Geometry check sheet. Reference: drawing and pictorial views, mm from the part's lowest x, y, z. A direction names the side the tool comes from. Round coordinates to 2 decimals unless told otherwise and drop trailing zeros. Order: outer loops, then holes, each group sorted by start corner. A loop starts at its lowest first (then second) coordinate and runs counter-clockwise, first axis right, second up.
Q1. Cross-section at B-B on x = 13.75. Record the cut outline in (y, z), then the cut area to 3 significant figures.
Q2. Cross-section at A-A on z = 8. Record the cut outline in (x, y).
Q3. Set-up check for the marked faces 5, 6, 7, 8 and 9: record each of +Z, -Z, +X, -X, +Y, -Y from which the full face is reachable in a straight line by a thin tool's end or side.
Q4. Cross-section at C-C on x = 2.5. Record the cut outline in (y, z).
Q5. Scan lines: probe 1 along Y at (x, z) = (11.75, 12); probe 2 along X at (y, z) = (10.5, 4); probe 3 along Z at (x, y) = (11.75, 5.25). Record each from-to range of solid material in increasing order.
Q6. Depth check by flat-ended pin: P1, Ø0.6, axis at x = 16, y = 2.5, coming from the +Z side; P2, Ø0.6, axis at x = 11, y = 6.5, coming from the +Z side; P3, Ø2.5, axis at x = 5, z = 8.5, coming from the -Y side. Enter the tip coordinate at first touch or a pass-through.
Q7. Cross-section at D-D on z = 4.25. Record the cut outline in (x, y).
Q8. Mould release check, pull along X, two halves, no side actions. Record for the marked faces 1, 2, 3 and 4: +X half, -X half, draft (parallel to the pull), parting line (faces both ways), or undercut.
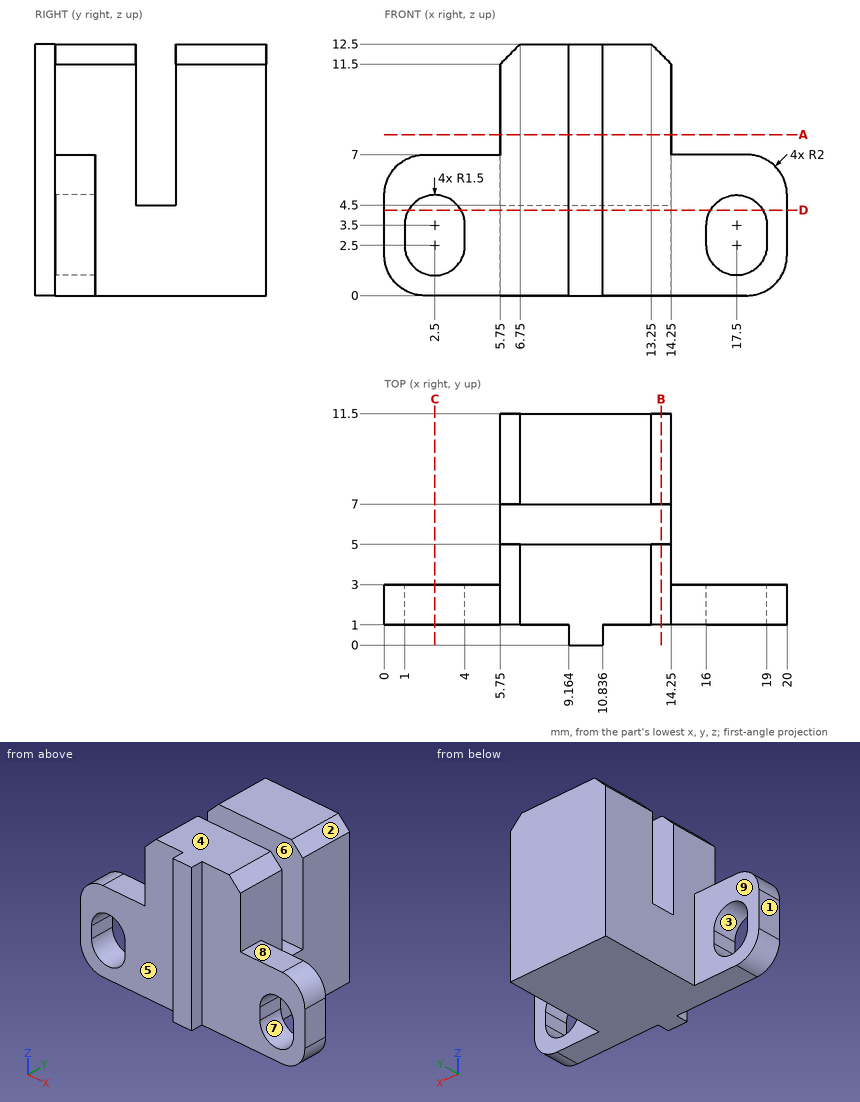
Results found:
1. outline: (1, 0) - (11.5, 0) - (11.5, 12) - (7, 12) - (7, 4.5) - (5, 4.5) - (5, 12) - (1, 12) - close
1. area: 111 mm2
2. outline: (5.75, 1) - (9.16, 1) - (9.16, 0) - (10.84, 0) - (10.84, 1) - (14.25, 1) - (14.25, 5) - (5.75, 5) - close; (5.75, 7) - (14.25, 7) - (14.25, 11.5) - (5.75, 11.5) - close
3. face 5: +Z, -Z, -X, -Y
3. face 6: +Z, +X, -X
3. face 7: +Y, -Y
3. face 8: +Z, +X, +Y, -Y
3. face 9: +Z, -Z, -X, +Y
4. outline: (1, 0) - (3, 0) - (3, 1) - (1, 1) - close; (1, 5) - (3, 5) - (3, 7) - (1, 7) - close
5. probe 1: y = 1 to 5, 7 to 11.5
5. probe 2: x = 5.75 to 14.25
5. probe 3: z = 0 to 4.5
6. P1: stops at z = 7
6. P2: stops at z = 4.5
6. P3: stops at y = 1
7. outline: (0, 1) - (1.2, 1) - (1.2, 3) - (0, 3) - close; (3.8, 1) - (9.16, 1) - (9.16, 0) - (10.84, 0) - (10.84, 1) - (16.2, 1) - (16.2, 3) - (14.25, 3) - (14.25, 11.5) - (5.75, 11.5) - (5.75, 3) - (3.8, 3) - close; (18.8, 1) - (20, 1) - (20, 3) - (18.8, 3) - close
8. face 1: -X half
8. face 2: +X half
8. face 3: undercut
8. face 4: draft
